```python
from build123d import *

# Parameters (mm, degrees)
SKETCH1_R           = 1.6
BOSS_EXTRUDE1_DEPTH = 5.9944


with BuildPart() as part:
    # Sketch1 → Boss-Extrude1 (new body)
    with BuildSketch(Plane.XY):
        with BuildLine():
            Line((-3.01403503, 3.046744767), (-31.75, 2.9972))
            Line((-31.75, 2.9972), (-37.7444, 2.9972))
            Line((-37.7444, 2.9972), (-42.403721744, 2.9972))
            Line((-42.403721744, 2.9972), (-61.453721744, 2.9972))
            Line((-61.453721744, 2.9972), (-61.453721744, -2.9972))
            Line((-61.453721744, -2.9972), (-55.103721744, -2.9972))
            Line((-55.103721744, -2.9972), (-42.403721744, -2.9972))
            Line((-42.403721744, -2.9972), (-37.7444, -2.9972))
            Line((-37.7444, -2.9972), (-31.75, -2.9972))
            Line((-31.75, -2.9972), (-3.01403503, -3.046744767))
            ThreePointArc((-3.01403503, -3.046744767), (-2.393607559, -3.124787196), (-1.8110486, -3.352044595))
            ThreePointArc((-1.8110486, -3.352044595), (3.81, 0), (-1.8110486, 3.352044595))
            ThreePointArc((-1.8110486, 3.352044595), (-2.393607559, 3.124787196), (-3.01403503, 3.046744767))
        make_face()
        with Locations((-27.94, 0)):
            Circle(SKETCH1_R, mode=Mode.SUBTRACT)
        Circle(SKETCH1_R, mode=Mode.SUBTRACT)
    extrude(amount=BOSS_EXTRUDE1_DEPTH)


solid = part.part
```
Work out the finished part from the listing and answer in its coordinate system (mm). A direction names the side the tool comes from. Give positions to 0.01 mm unless a question says otherwise; leave off trailing zeros. Loops run counter-clockwise (first coordinate to the right, second up) from the corner with the lowest first, then second, coordinate; pieces in that order, holes last. Notation, with made-up numbers: (-26, -4.5) -> (3, -4.5) arc R25 cw to (3, 33.5) -> close; hole circle Ø1 at (-4, -18). An arc over 180 degrees is marked (long way). One line per question, with ' | ' between items. Start each with the question number.
1) Section B-B, the plane y = 0 is taken. Determine the outline of the cut face in (x, z), then the cut area to 3 significant figures.
2) Section A-A, the plane x = 0 is taken. Determine the outline of the cut face in (y, z).
3) For faces 1 (the face through (-2.385, 3.127, 2.955)), 2 (the face through (-47, -2.997, 3)), determine the directions among +Z, -Z, +X, -X, +Y, -Y from which every point of the face is accessible in a straight line to the end or side of a thin tool.
4) Straight lines are drawn through the part: L1, parallel to Y at x = -27.94, z = 4.65; L2, parallel to Y at x = 0, z = 4.6; L3, parallel to X at y = 0.25, z = 1.5. For each, find the intervals that lie inside material, in ascending order.
5) Determine the mould class of faces 3 (the face through (-29.54, 0.07, 2.96)), 4 (the face through (-1.27, -0.97, 2.96)), 5 (the face through (-46, 2.997, 3)), 6 (the face through (-61.454, 0, 3)) for opening direction X: +X half, -X half, draft (parallel to the pull), parting line (faces both ways), or undercut.
6) Each of these flat-tipped pins is pushed along its axis until it touches: pin 1 (3.5 mm diameter, centred on x = 0, y = 0, fed in from +Z); pin 2 (1.5 mm diameter, centred on y = 2.5, z = 5.5, fed in from +X); pin 3 (3 mm diameter, centred on y = -2.5, z = 3.5, fed in from +X). Where does it stop, or does it pass through?
7) Section D-D, the plane x = -27.94 is taken. Determine the outline of the cut face in (y, z), then the cut area to 3 significant figures.
8) Section C-C, the plane z = 3.45 is taken. Determine the outline of the cut face in (x, y), then the cut area to 3 significant figures.
Resolved:
1) outline: (-61.45, 0) -> (-29.54, 0) -> (-29.54, 5.99) -> (-61.45, 5.99) -> close; (-26.34, 0) -> (-1.6, 0) -> (-1.6, 5.99) -> (-26.34, 5.99) -> close; (1.6, 0) -> (3.81, 0) -> (3.81, 5.99) -> (1.6, 5.99) -> close | area: 353 mm2
2) outline: (-3.81, 0) -> (-1.6, 0) -> (-1.6, 5.99) -> (-3.81, 5.99) -> close; (1.6, 0) -> (3.81, 0) -> (3.81, 5.99) -> (1.6, 5.99) -> close
3) face 1: +Z, -Z, -X, +Y | face 2: +Z, -Z, -X, -Y
4) L1: -3 to -1.6, 1.6 to 3 | L2: -3.81 to -1.6, 1.6 to 3.81 | L3: -61.45 to -29.52, -26.36 to -1.58, 1.58 to 3.8
5) face 3: undercut | face 4: undercut | face 5: draft | face 6: -X half
6) pin 1: z = 5.99 | pin 2: x = 3.38 | pin 3: x = 3.68
7) outline: (-3, 0) -> (-1.6, 0) -> (-1.6, 5.99) -> (-3, 5.99) -> close; (1.6, 0) -> (3, 0) -> (3, 5.99) -> (1.6, 5.99) -> close | area: 16.8 mm2
8) outline: (-61.45, -3) -> (-31.75, -3) -> (-3.01, -3.05) arc R2.54 cw to (-1.81, -3.35) arc R3.81 ccw (long way) to (-1.81, 3.35) arc R2.54 cw to (-3.01, 3.05) -> (-31.75, 3) -> (-61.45, 3) -> close; hole circle Ø3.2 at (-27.94, 0); hole circle Ø3.2 at (0, 0) | area: 379 mm2
